Build history of the part. All positions in model axes, mm. Face numbers are marked on the shaded views. A direction names the side the tool comes from. Round coordinates to 2 decimals unless told otherwise and drop trailing zeros. Write each loop counter-clockwise with the first axis right and the second up, starting at its lowest first coordinate (ties: lowest second). Pieces come first, ordered by that corner, then holes. Notation, with made-up numbers: (14.25, 51) -> (29.25, 51) arc R27 ccw to (29.25, 71) -> close; hole circle Ø7 at (58, 63). An arc over 180 degrees is marked (long way). Return JSON: item names as keys, results as strings.
Solid Edge part; units mm, degrees
sketch "Sketch1" plane through (0, 0, 0) normal (0, 0, 1) x (1, 0, 0)
  circle A0 centre (0, 0) radius 35
extrude "Protrusion1" add sketch "Sketch1" against normal blind 38.5823
hole "Hole_3" at (0, 0, 0) direction (0, 0, -1) diameter 60 depth 30
sketch "Sketch2" plane through (26.5265, -22.833, -19.2912) normal (0.7579, -0.6524, 0) x (0, 0, 1)
  line L0 (-6.0379, 0.3201) -> (0.9621, 0.3201)
  line L1 (0.9621, 0.3201) -> (0.9621, 10.3801)
  line L2 (0.9621, 10.3801) -> (-6.0379, 10.3801)
  line L3 (-6.0379, 10.3801) -> (-6.0379, 0.3201)
extrude "Protrusion2" add sketch "Sketch2" against normal blind 1.6301
properties material "Galvanized steel"
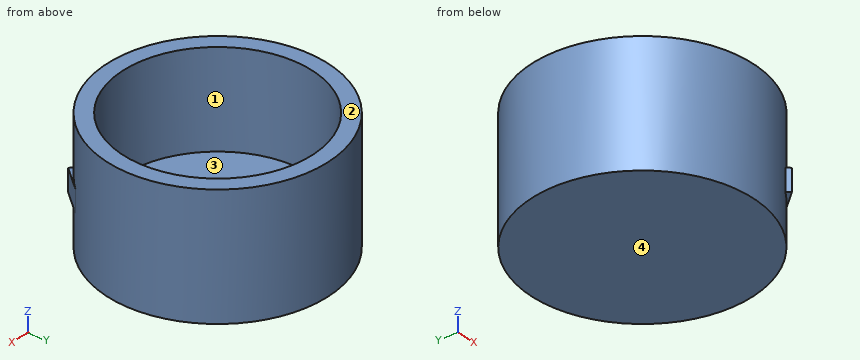
Q1. Wall check: L1, parallel to Y at x = 0, z = -9; L2, parallel to Z at x = 16, y = 5.5; L3, parallel to Y at x = 4, z = -3. Give the ranges that are in metal, low to high.
Verdict:
{"L1": "y = -35 to -30, 30 to 35", "L2": "z = -38.58 to -30", "L3": "y = -34.77 to -29.73, 29.73 to 34.77"}
Q2. Pin check, flat tips, straight feed: pin 1 Ø10 at (y, z) = (11.5, -8.5) entering from +X; pin 2 Ø12 at (x, y) = (1.5, 15) entering from +Z; pin 3 Ø5 at (x, z) = (15, -21.5) entering from +Y; pin 4 Ø2.5 at (x, y) = (24, -25.5) entering from +Z. Stop position of each tip, or through.
Verdict:
{"pin 1": "stops at x = 34.39", "pin 2": "stops at z = -30", "pin 3": "stops at y = 32.69", "pin 4": "stops at z = 0"}
Q3. Saw through at B-B on y = 0. List the corners of the cut face in (x, z).
Verdict:
{"outline": "(-35, -38.58) -> (35, -38.58) -> (35, 0) -> (30, 0) -> (30, -30) -> (-30, -30) -> (-30, 0) -> (-35, 0) -> close"}
Q4. Saw through at D-D on z = -13. List the corners of the cut face in (x, y), then the cut area to 3 significant figures.
Verdict:
{"outline": "circle Ø70 at (0, 0); hole circle Ø60 at (0, 0)", "area": "1,020 mm²"}
Q5. 3-axis set-ups, long thin cutter, end or side, ignore diameter. For the marked faces 3 and 4: which of +Z, -Z, +X, -X, +Y, -Y reach the whole face in a straight line?
Verdict:
{"face 3": "+Z", "face 4": "-Z, +X, -X, +Y, -Y"}
Q6. Saw through at C-C on x = -7. List the corners of the cut face in (y, z).
Verdict:
{"outline": "(-34.29, -38.58) -> (34.29, -38.58) -> (34.29, 0) -> (29.17, 0) -> (29.17, -30) -> (-29.17, -30) -> (-29.17, 0) -> (-34.29, 0) -> close"}
Q7. Two-plate mould, pull along X, no slides. Class the marked faces 1 and 2: +X half, -X half, draft (parallel to the pull), parting line (faces both ways), or undercut.
Verdict:
{"face 1": "undercut", "face 2": "draft"}
